Autodesk Inventor part; units mm, degrees
ref_plane "YZ Plane" through (0, 0, 0) normal (1, 0, 0) x (0, 1, 0)
ref_plane "XZ Plane" through (0, 0, 0) normal (0, 1, 0) x (-1, 0, 0)
ref_plane "XY Plane" through (0, 0, 0) normal (0, 0, 1) x (1, 0, 0)
sketch "Sketch1" plane through (0, 0, 0) normal (0, 1, 0) x (-1, 0, 0)
  circle A0 centre (0, 0) radius 6.35
  circle A1 centre (0, 0) radius 1.5875
  dimension "d0" = 12.7
  dimension "d1" = 3.175
extrude "Extrusion1" add sketch "Sketch1" along normal blind 6.35 contours A1
thread "Thread1"
sketch "Sketch3" plane through (0, 6.35, 0) normal (0, 1, 0) x (1, 0, 0)
  line L0 (-2.6555, -1.6362) -> (-2.7448, 1.4816)
  line L1 (-2.7448, 1.4816) -> (-0.0893, 3.1178)
  line L2 (-0.0893, 3.1178) -> (2.6555, 1.6362)
  line L3 (2.6555, 1.6362) -> (2.7448, -1.4816)
  line L4 (2.7448, -1.4816) -> (0.0893, -3.1178)
  line L5 (0.0893, -3.1178) -> (-2.6555, -1.6362)
  point P0 (0, 0)
  point P1 (0, 0)
extrude "Extrusion3" add sketch "Sketch3" along normal blind 0.508
properties part number ".125bolt"
Design review of the part built by this model. Coordinates are the model's own, in mm. A direction names the side the tool comes from. Coordinates: 2 decimals unless noted, no trailing zeros. Write each loop counter-clockwise with the first axis right and the second up, starting at its lowest first coordinate (ties: lowest second). Pieces come first, ordered by that corner, then holes. Notation, with made-up numbers: (25, 56.25) - (77, 56.25) arc R14 cw to (77, 67.25) - close; hole circle Ø8 at (-35, 26.5). An arc over 180 degrees is marked (long way). One line per item, written item: value.
1) For faces 1 (the face through (1.436, 6.6, 2.288)), 2 (the face through (0.34, 3.13, 1.55)), list the 3-axis set-ups (+Z, -Z, +X, -X, +Y, -Y) from which the entire face can be reached by the end or side of a thin tool; tool diameter is ignored.
Answer sheet:
face 1: +Z, +X, +Y, -Y
face 2: -Y
2) To check wall thickness, follow probe 1 along Y at (x, z) = (-2.35, 1.25); probe 2 along X at (y, z) = (3.5, -1); probe 3 along X at (y, z) = (2, 1.25). State the ranges of each line that lie inside material, in increasing order.
Answer sheet:
probe 1: y = 6.35 to 6.86
probe 2: x = -1.23 to 1.23
probe 3: x = -0.98 to 0.98
3) Add section A-A (z = 1.25). State the section outline as (x, y) points.
Answer sheet:
outline: (-2.67, 6.35) - (-0.98, 6.35) - (-0.98, 0) - (0.98, 0) - (0.98, 6.35) - (2.74, 6.35) - (2.74, 6.86) - (-2.67, 6.86) - close
4) Add section B-B (x = -0.85). State the section outline as (y, z) points.
Answer sheet:
outline: (0, -1.34) - (6.35, -1.34) - (6.35, -2.65) - (6.86, -2.65) - (6.86, 2.61) - (6.35, 2.61) - (6.35, 1.34) - (0, 1.34) - close
5) Add section C-C (y = 6.5). State the section outline as (x, z) points.
Answer sheet:
outline: (-2.74, -1.48) - (-0.09, -3.12) - (2.66, -1.64) - (2.74, 1.48) - (0.09, 3.12) - (-2.66, 1.64) - close
6) Insertion check: pin 1 (3 mm diameter, centred on y = 1, z = 1, fed in from +X); pin 2 (3 mm diameter, centred on y = 3.5, z = 1, fed in from -X). Each pin has a flat end and moves straight along its axis. Give the tip position at first contact, or say it passes through.
Answer sheet:
pin 1: stops at x = 1.59
pin 2: stops at x = -1.59
7) Add section D-D (x = -2). State the section outline as (y, z) points, plus the area to 3 significant figures.
Answer sheet:
outline: (6.35, -1.94) - (6.86, -1.94) - (6.86, 1.99) - (6.35, 1.99) - close
area: 2.00 mm2
